from build123d import *

# Parameters (mm, degrees)
F0_R     = 42.5
F0_R_2   = 1.65
F0_R_3   = 30.75
F1_DEPTH = 16
F2_R     = 42.5
F2_R_2   = 1.65
F2_R_3   = 26.5
F3_DEPTH = 2


with BuildPart() as f1:
    # F0 (on Top) → F1 (new body)
    with BuildSketch(Plane.XY):
        Circle(F0_R)
        with Locations((0, -38)):
            Circle(F0_R_2, mode=Mode.SUBTRACT)
        with Locations((-38, 0)):
            Circle(F0_R_2, mode=Mode.SUBTRACT)
        Circle(F0_R_3, mode=Mode.SUBTRACT)
        with Locations((38, 0)):
            Circle(F0_R_2, mode=Mode.SUBTRACT)
        with Locations((0, 38)):
            Circle(F0_R_2, mode=Mode.SUBTRACT)
    extrude(amount=F1_DEPTH)

    # F2 (on Top) → F3 (join)
    with BuildSketch(Plane.XY):
        Circle(F2_R)
        with Locations((0, -38)):
            Circle(F2_R_2, mode=Mode.SUBTRACT)
        with Locations((-38, 0)):
            Circle(F2_R_2, mode=Mode.SUBTRACT)
        Circle(F2_R_3, mode=Mode.SUBTRACT)
        with Locations((38, 0)):
            Circle(F2_R_2, mode=Mode.SUBTRACT)
        with Locations((0, 38)):
            Circle(F2_R_2, mode=Mode.SUBTRACT)
    extrude(amount=-F3_DEPTH)


solid = f1.part
Could you check a few things on this model? Use its own coordinates, in mm. A direction names the side the tool comes from. Give positions to 0.01 mm unless a question says otherwise; leave off trailing zeros. Order: outer loops, then holes, each group sorted by start corner. A loop starts at its lowest first (then second) coordinate and runs counter-clockwise, first axis right, second up. Notation, with made-up numbers: (-35.5, -12) - (9.5, -12) arc R25 ccw to (9.5, 27) - close; hole circle Ø8 at (82, -7.5). An arc over 180 degrees is marked (long way). Return JSON: item names as keys, results as strings. Group by question number.
Q1. Please list where these lines run through material, in increasing order: line 1 along Y through (x, z) = (0, -1.45); line 2 along Y through (x, z) = (0, 12.25); line 3 along Y through (x, z) = (4.5, 4.75). Write a range as [from, to].
Q2. Will these pins go through, and if not, where does the flat tip stop? pin 1 Ø3 at (x, y) = (0, -38) entering from -Z; pin 2 Ø3 at (x, z) = (-8.5, 0) entering from +Y; pin 3 Ø4 at (y, z) = (-17.5, 5) entering from -X; pin 4 Ø3 at (x, z) = (21.5, 6.5) entering from +Y.
Q3. Which directions (+Z, -Z, +X, -X, +Y, -Y) give clear straight access to the entire face, cutting with the end or side of a thin tool? Please do faces 1 (the face through (-39.65, 0.07, 6.87)), 2 (the face through (9, 25.2, 0)).
Q4. Suppose I cut it at A-A, the plane y = 0. Please give me the cut outline in (x, z).
Q5. Thinking about a two-plate mould opening in Y: for faces 3 (the face through (-19.5, -18.3, -2)), 4 (the face through (-33.727, -25.861, 7.126)), 5 (the face through (14.19, -27.28, 7.89)), 6 (the face through (0.89, -36.61, 6.87)), which applies, pulls with the +Y half, pulls with the -Y half, needs draft (parallel to the pull), parting line crosses it, or undercut?
Q6. Suppose I cut it at C-C, the plane z = 8. Please give me the cut outline in (x, y), and give its area (3 significant figures).
Q7. Suppose I cut it at D-D, the plane x = 38. Please give me the cut outline in (y, z), and give its area (3 significant figures).
Resolved:
{
 "1": {"line 1": "y = [-42.5, -39.65], [-36.35, -26.5], [26.5, 36.35], [39.65, 42.5]", "line 2": "y = [-42.5, -39.65], [-36.35, -30.75], [30.75, 36.35], [39.65, 42.5]", "line 3": "y = [-42.26, -30.42], [30.42, 42.26]"},
 "2": {"pin 1": "passes through", "pin 2": "stops at y = 41.92", "pin 3": "stops at x = -39.57", "pin 4": "stops at y = 37.5"},
 "3": {"face 1": "+Z, -Z", "face 2": "+Z"},
 "4": {"outline": "(-42.5, -2) - (-39.65, -2) - (-39.65, 16) - (-42.5, 16) - close; (-36.35, -2) - (-26.5, -2) - (-26.5, 0) - (-30.75, 0) - (-30.75, 16) - (-36.35, 16) - close; (26.5, -2) - (36.35, -2) - (36.35, 16) - (30.75, 16) - (30.75, 0) - (26.5, 0) - close; (39.65, -2) - (42.5, -2) - (42.5, 16) - (39.65, 16) - close"},
 "5": {"face 3": "needs draft", "face 4": "parting line crosses it", "face 5": "undercut", "face 6": "undercut"},
 "6": {"outline": "circle Ø85 at (0, 0); hole circle Ø3.3 at (-38, 0); hole circle Ø61.5 at (0, 0); hole circle Ø3.3 at (0, -38); hole circle Ø3.3 at (0, 38); hole circle Ø3.3 at (38, 0)", "area": "2,670 mm2"},
 "7": {"outline": "(-19.03, -2) - (-1.65, -2) - (-1.65, 16) - (-19.03, 16) - close; (1.65, -2) - (19.03, -2) - (19.03, 16) - (1.65, 16) - close", "area": "626 mm2"}
}
